```python
from build123d import *

# Parameters (mm, degrees)
F0_W     = 40
F0_H     = 42
F0_W_2   = 36
F0_H_2   = 10.092967
F0_W_3   = 13.144892
F0_H_3   = 25.934145
F0_W_4   = 21.089894
F1_DEPTH = 70
F4_DEPTH = 2


with BuildPart() as f1:
    # F0 (on Front) → F1 (new body)
    with BuildSketch(Plane.XZ):
        with Locations((90.064679, 37.446823)):
            Rectangle(F0_W, F0_H)
        with Locations((90.064679, 23.493306)):
            Rectangle(F0_W_2, F0_H_2, mode=Mode.SUBTRACT)
        with Locations((78.637125, 43.47975)):
            Rectangle(F0_W_3, F0_H_3, mode=Mode.SUBTRACT)
        with Locations((97.519732, 43.47975)):
            Rectangle(F0_W_4, F0_H_3, mode=Mode.SUBTRACT)
    extrude(amount=-F1_DEPTH)

    # F3 (on face) → F4 (join)
    with BuildSketch(Plane.XZ):
        Polygon((110.064679, 62.446823), (66.064679, 62.446823), (66.064679, 16.446823), (70.064679, 16.446823), (70.064679, 58.446823), (110.064679, 58.446823), align=None)
    extrude(amount=-F4_DEPTH)


solid = f1.part
```
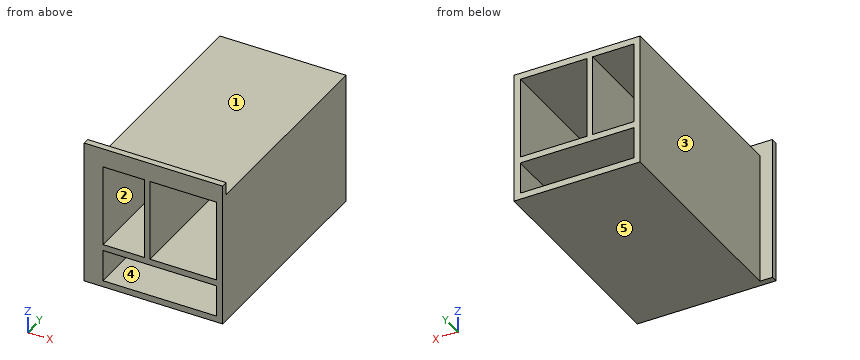
The model under review builds one solid part; all positions refer to its coordinate system, in mm. Face numbers are marked on the shaded views. A direction names the side the tool comes from. Coordinates: 2 decimals unless noted, no trailing zeros. Order: outer loops, then holes, each group sorted by start corner. A loop starts at its lowest first (then second) coordinate and runs counter-clockwise, first axis right, second up. Notation, with made-up numbers: (-1.75, 25.25) -> (9.25, 25.25) arc R21 ccw to (9.25, 55.25) -> close; hole circle Ø3 at (11.5, -5.75). An arc over 180 degrees is marked (long way). Answer in a Markdown table with one row per item. Add a question column.
Item 1: Machinability: for the marked faces 4 and 5, which of the approach directions +Z, -Z, +X, -X, +Y, -Y give a long, thin tool a straight path to every point of the face, cutting with its end or side? Answer none if there is none.
Item 2: Clearance check with flat-ended pins moving along their axes: pin 1 (10.5 mm diameter, centred on x = 76.5, y = 27, fed in from +Z); pin 2 (4 mm diameter, centred on x = 105, z = 44.5, fed in from +Y); pin 3 (6 mm diameter, centred on y = 26, z = 23.5, fed in from -X). State where each tip first meets the part, or that it passes through.
Item 3: We need section A-A on x = 94. Write out the cut boundary in (y, z), plus the area to 3 significant figures.
Item 4: Mouldability with a two-part tool opening along Z and no side actions: class the marked faces 1, 2 and 3 as +Z half, -Z half, draft (parallel to the pull), parting line (faces both ways), or undercut.
Item 5: We need section D-D on z = 23. Write out the cut boundary in (x, y).
Item 6: We need section C-C on y = 10. Write out the cut boundary in (x, z).
Item 7: We need section B-B on z = 34.5. Write out the cut boundary in (x, y).
Item 8: To check wall thickness, follow probe 1 along X at (y, z) = (61.5, 44.5); probe 2 along Z at (x, y) = (75.5, 55.5); probe 3 along X at (y, z) = (5, 28). State the ranges of each line that lie inside material, in increasing order.
Final values:
| question | item | result |
|---|---|---|
| 1 | face 4 | +Y, -Y |
| 1 | face 5 | -Z, +X, -X, +Y, -Y |
| 2 | pin 1 | stops at z = 58.45 |
| 2 | pin 2 | passes through |
| 2 | pin 3 | stops at x = 70.06 |
| 3 | outline | (0, 16.45) -> (70, 16.45) -> (70, 18.45) -> (0, 18.45) -> close; (0, 28.54) -> (70, 28.54) -> (70, 30.51) -> (0, 30.51) -> close; (0, 56.45) -> (70, 56.45) -> (70, 58.45) -> (2, 58.45) -> (2, 62.45) -> (0, 62.45) -> close |
| 3 | area | 426 mm2 |
| 4 | face 1 | +Z half |
| 4 | face 2 | undercut |
| 4 | face 3 | draft |
| 5 | outline | (66.06, 0) -> (72.06, 0) -> (72.06, 70) -> (70.06, 70) -> (70.06, 2) -> (66.06, 2) -> close; (108.06, 0) -> (110.06, 0) -> (110.06, 70) -> (108.06, 70) -> close |
| 6 | outline | (70.06, 16.45) -> (110.06, 16.45) -> (110.06, 58.45) -> (70.06, 58.45) -> close; hole (72.06, 18.45) -> (108.06, 18.45) -> (108.06, 28.54) -> (72.06, 28.54) -> close; hole (72.06, 30.51) -> (85.21, 30.51) -> (85.21, 56.45) -> (72.06, 56.45) -> close; hole (86.97, 30.51) -> (108.06, 30.51) -> (108.06, 56.45) -> (86.97, 56.45) -> close |
| 7 | outline | (66.06, 0) -> (72.06, 0) -> (72.06, 70) -> (70.06, 70) -> (70.06, 2) -> (66.06, 2) -> close; (85.21, 0) -> (86.97, 0) -> (86.97, 70) -> (85.21, 70) -> close; (108.06, 0) -> (110.06, 0) -> (110.06, 70) -> (108.06, 70) -> close |
| 8 | probe 1 | x = 70.06 to 72.06, 85.21 to 86.97, 108.06 to 110.06 |
| 8 | probe 2 | z = 16.45 to 18.45, 28.54 to 30.51, 56.45 to 58.45 |
| 8 | probe 3 | x = 70.06 to 72.06, 108.06 to 110.06 |
